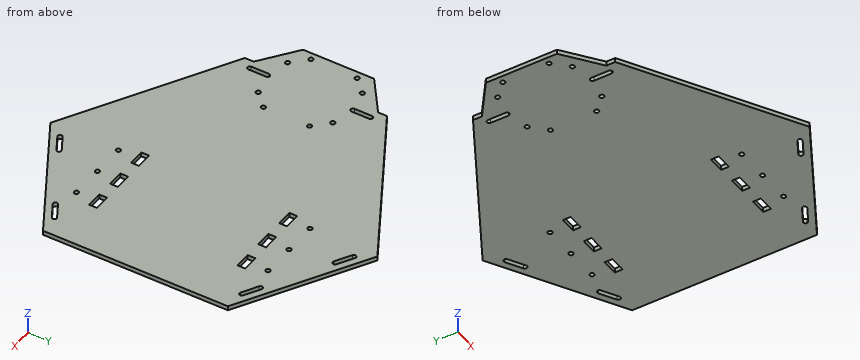
```python
from build123d import *

# Parameters (mm, degrees)
F1_DEPTH = 3.175
F2_R     = 1.5875
F2_W     = 11.43
F2_H     = 5.588
F3_DEPTH = 25.4


with BuildPart() as f1:
    # F0 (on Top) → F1 (new body)
    with BuildSketch(Plane.XY):
        Polygon((-79.823994, 0), (-105.223994, -19.05), (-105.223994, -69.85), (-79.823994, -88.9), (-79.823994, -95.25), (34.560641, -161.29), (122.548823, -110.49), (122.548823, 21.59), (34.560641, 72.39), (-79.823994, 6.35), align=None)
    extrude(amount=F1_DEPTH)

    # F2 (on face) → F3 (cut)
    with BuildSketch(Plane.XY.offset(3.175)):
        with Locations((-100.143994, -27.94)):
            Circle(F2_R)
        with Locations((-89.983994, -17.78)):
            Circle(F2_R)
        with Locations((-56.963994, -17.78)):
            Circle(F2_R)
        with Locations((-46.803994, -27.94)):
            Circle(F2_R)
        with Locations((-46.803994, -60.96)):
            Circle(F2_R)
        with Locations((-56.963994, -71.12)):
            Circle(F2_R)
        with Locations((-89.983994, -71.12)):
            Circle(F2_R)
        with Locations((-100.143994, -60.96)):
            Circle(F2_R)
        with BuildLine():
            Line((-75.061494, -74.93), (-75.061494, -87.63))
            ThreePointArc((-75.061494, -87.63), (-73.473994, -89.2175), (-71.886494, -87.63))
            Line((-71.886494, -87.63), (-71.886494, -74.93))
            ThreePointArc((-71.886494, -74.93), (-73.473994, -73.3425), (-75.061494, -74.93))
        make_face()
        with BuildLine():
            Line((-71.886494, -13.97), (-71.886494, -1.27))
            ThreePointArc((-71.886494, -1.27), (-73.473994, 0.3175), (-75.061494, -1.27))
            Line((-75.061494, -1.27), (-75.061494, -13.97))
            ThreePointArc((-75.061494, -13.97), (-73.473994, -15.5575), (-71.886494, -13.97))
        make_face()
        with Locations((34.283823, 8.509)):
            Rectangle(F2_W, F2_H)
        with Locations((57.778823, 8.509)):
            Rectangle(F2_W, F2_H)
        with Locations((81.273823, 8.509)):
            Rectangle(F2_W, F2_H)
        with Locations((57.778823, 24.003)):
            Circle(F2_R)
        with Locations((34.283823, 24.003)):
            Circle(F2_R)
        with Locations((81.273823, -97.409)):
            Rectangle(F2_W, F2_H)
        with Locations((57.778823, -97.409)):
            Rectangle(F2_W, F2_H)
        with Locations((34.283823, -97.409)):
            Rectangle(F2_W, F2_H)
        with Locations((34.283823, -112.903)):
            Circle(F2_R)
        with Locations((57.778823, -112.903)):
            Circle(F2_R)
        with Locations((81.273823, -112.903)):
            Circle(F2_R)
        with BuildLine():
            ThreePointArc((109.16905, -112.715554), (107.000485, -112.134489), (107.58155, -109.965923))
            Line((107.58155, -109.965923), (96.583027, -116.315923))
            ThreePointArc((96.583027, -116.315923), (98.170527, -116.315923), (98.964277, -117.690739))
            ThreePointArc((98.964277, -117.690739), (98.751593, -118.484489), (98.170527, -119.065554))
            Line((98.170527, -119.065554), (109.16905, -112.715554))
        make_face()
        with BuildLine():
            ThreePointArc((98.964277, -117.690739), (98.170527, -116.315923), (96.583027, -116.315923))
            ThreePointArc((96.583027, -116.315923), (96.001962, -118.484489), (98.170527, -119.065554))
            ThreePointArc((98.170527, -119.065554), (98.751593, -118.484489), (98.964277, -117.690739))
        make_face()
        with BuildLine():
            ThreePointArc((109.16905, -112.715554), (109.750115, -112.134489), (109.9628, -111.340739))
            ThreePointArc((109.9628, -111.340739), (109.16905, -109.965923), (107.58155, -109.965923))
            ThreePointArc((107.58155, -109.965923), (107.000485, -112.134489), (109.16905, -112.715554))
        make_face()
        with BuildLine():
            Line((52.588937, -141.715923), (41.590414, -148.065923))
            ThreePointArc((41.590414, -148.065923), (41.009349, -150.234489), (43.177914, -150.815554))
            Line((43.177914, -150.815554), (54.176437, -144.465554))
            ThreePointArc((54.176437, -144.465554), (54.757502, -142.296989), (52.588937, -141.715923))
        make_face()
        with BuildLine():
            Line((96.583027, 27.415923), (107.58155, 21.065923))
            ThreePointArc((107.58155, 21.065923), (109.750115, 21.646989), (109.16905, 23.815554))
            Line((109.16905, 23.815554), (98.170527, 30.165554))
            ThreePointArc((98.170527, 30.165554), (96.001962, 29.584489), (96.583027, 27.415923))
        make_face()
        with BuildLine():
            Line((54.176437, 55.565554), (43.177914, 61.915554))
            ThreePointArc((43.177914, 61.915554), (41.009349, 61.334489), (41.590414, 59.165923))
            Line((41.590414, 59.165923), (52.588937, 52.815923))
            ThreePointArc((52.588937, 52.815923), (54.757502, 53.396989), (54.176437, 55.565554))
        make_face()
        with Locations((81.273823, 24.003)):
            Circle(F2_R)
    extrude(amount=-F3_DEPTH, mode=Mode.SUBTRACT)


solid = f1.part
```
Geometry: final body of the model. Coordinates: model frame, mm. Round coordinates to 2 decimals unless told otherwise and drop trailing zeros. Order: outer loops, then holes, each group sorted by start corner. A loop starts at its lowest first (then second) coordinate and runs counter-clockwise, first axis right, second up. Notation, with made-up numbers: (74.25, 72) -> (100.25, 72) arc R19 ccw to (100.25, 98) -> close; hole circle Ø11 at (0, 73.5). An arc over 180 degrees is marked (long way). Use one line per item in the form item = value. Start each with the question number.
1. Pin query (flat end, axial travel): pin 1 Ø4 at (x, y) = (-89.98, -71.12) entering from +Z (3 decimals); pin 2 Ø2.5 at (x, y) = (-56.96, -71.12) entering from -Z; pin 3 Ø1.6 at (x, z) = (36, 1) entering from -Y; pin 4 Ø1 at (x, z) = (82, 1.5) entering from -Y. Return the tip coordinate at first contact, or that it passes through.
2. Cut plane C-C (x = -5). Return the cut outline in (y, z) (3 decimals), then the cut area to 3 significant figures.
3. Cut plane A-A (x = 48). Return the cut outline in (y, z) (3 decimals), then the cut area to 3 significant figures.
4. Cut plane B-B (y = 36). Return the cut outline in (x, z) (3 decimals).
5. Cut plane D-D (z = 0.85). Count the separate pieces of the cut face and the enclosed holes in it, then the cut area to 3 significant figures.
6. Line query: probe 1 along X at (y, z) = (-98, 1.9); probe 2 along Y at (x, z) = (50, 1.6); probe 3 along X at (y, z) = (-114, 0.5). Output: solid intervals per line, ascending.
Solution:
q1.pin_1 = 3.175
q1.pin_2 = through
q1.pin_3 = -160.92
q1.pin_4 = -134.19
q2.outline = (-138.45, 0) -> (49.55, 0) -> (49.55, 3.175) -> (-138.45, 3.175) -> close
q2.area = 597 mm^2
q3.outline = (-153.531, 0) -> (-148.032, 0) -> (-148.032, 3.175) -> (-153.531, 3.175) -> close; (-144.365, 0) -> (55.465, 0) -> (55.465, 3.175) -> (-144.365, 3.175) -> close; (59.132, 0) -> (64.631, 0) -> (64.631, 3.175) -> (59.132, 3.175) -> close
q3.area = 669 mm^2
q4.outline = (-28.469, 0) -> (97.59, 0) -> (97.59, 3.175) -> (-28.469, 3.175) -> close
q5.separate_pieces = 1
q5.enclosed_holes = 26
q5.area = 36,300 mm^2
q6.probe_1 = -75.06 to 28.57, 40 to 52.06, 63.49 to 75.56, 86.99 to 122.55
q6.probe_2 = -152.38 to -146.88, -143.21 to 54.31, 57.98 to 63.48
q6.probe_3 = -47.35 to 33.14, 35.43 to 56.63, 58.93 to 80.13, 82.42 to 100.59, 106.94 to 116.47
